```python
from build123d import *

# Parameters (mm, degrees)
BOSS_EXTRU_1_DEPTH = 10


with BuildPart() as part:
    # Esquisse1 → Boss.-Extru.1 (new body)
    with BuildSketch(Plane.XY):
        with BuildLine():
            Line((19.936371996, 9.53093454), (18.936003853, 6.945485686))
            ThreePointArc((18.936003853, 6.945485686), (18.933149277, 6.736662361), (19.067266911, 6.576575542))
            Line((19.067266911, 6.576575542), (21.475916438, 5.204099801))
            ThreePointArc((21.475916438, 5.204099801), (21.716214662, 4.879285253), (21.63795919, 4.482896797))
            Line((21.63795919, 4.482896797), (20.047921516, 2.211980154))
            ThreePointArc((20.047921516, 2.211980154), (19.995175197, 2.009908), (20.087084333, 1.822376562))
            Line((20.087084333, 1.822376562), (22.097287938, -0.08664509))
            ThreePointArc((22.097287938, -0.08664509), (22.252870323, -0.459528247), (22.082026846, -0.825670614))
            Line((22.082026846, -0.825670614), (19.994726852, -2.650077625))
            ThreePointArc((19.994726852, -2.650077625), (19.895154214, -2.833654908), (19.939513426, -3.03773232))
            Line((19.939513426, -3.03773232), (21.434445383, -5.372354483))
            ThreePointArc((21.434445383, -5.372354483), (21.496270047, -5.771635635), (21.242767367, -6.08625305))
            Line((21.242767367, -6.08625305), (18.779511342, -7.358122524))
            ThreePointArc((18.779511342, -7.358122524), (18.638899183, -7.512536093), (18.633130477, -7.72129924))
            Line((18.633130477, -7.72129924), (19.525910774, -10.345842161))
            ThreePointArc((19.525910774, -10.345842161), (19.490384691, -10.748316538), (19.168955462, -10.993124582))
            Line((19.168955462, -10.993124582), (16.472898893, -11.638540088))
            ThreePointArc((16.472898893, -11.638540088), (16.299419082, -11.754815988), (16.243857712, -11.956132315))
            Line((16.243857712, -11.956132315), (16.482601205, -14.718067098))
            ThreePointArc((16.482601205, -14.718067098), (16.351789022, -15.100344354), (15.981113543, -15.261115671))
            Line((15.981113543, -15.261115671), (13.208941437, -15.242568007))
            ThreePointArc((13.208941437, -15.242568007), (13.01267599, -15.313948704), (12.910550982, -15.496118438))
            Line((12.910550982, -15.496118438), (12.481382765, -18.234931474))
            ThreePointArc((12.481382765, -18.234931474), (12.262886811, -18.574795043), (11.864507393, -18.642186189))
            Line((11.864507393, -18.642186189), (9.177328317, -17.960753277))
            ThreePointArc((9.177328317, -17.960753277), (8.969683468, -17.983090385), (8.826929956, -18.135526484))
            Line((8.826929956, -18.135526484), (7.754791727, -20.692047914))
            ThreePointArc((7.754791727, -20.692047914), (7.461310193, -20.96974616), (7.0583792, -20.939840607))
            Line((7.0583792, -20.939840607), (4.612362234, -19.635124852))
            ThreePointArc((4.612362234, -19.635124852), (4.405405547, -19.607120219), (4.230319846, -19.720963651))
            Line((4.230319846, -19.720963651), (2.577520381, -21.946617741))
            ThreePointArc((2.577520381, -21.946617741), (2.226109347, -22.146011853), (1.842043663, -22.020547603))
            Line((1.842043663, -22.020547603), (-0.220657578, -20.168374341))
            ThreePointArc((-0.220657578, -20.168374341), (-0.414898532, -20.091655495), (-0.612141077, -20.160290093))
            Line((-0.612141077, -20.160290093), (-2.74954708, -21.925729918))
            ThreePointArc((-2.74954708, -21.925729918), (-3.138464883, -22.035231834), (-3.481344755, -21.821500413))
            Line((-3.481344755, -21.821500413), (-5.040853572, -19.529511222))
            ThreePointArc((-5.040853572, -19.529511222), (-5.211090216, -19.408536784), (-5.419026585, -19.427973754))
            Line((-5.419026585, -19.427973754), (-7.91682086, -20.630598369))
            ThreePointArc((-7.91682086, -20.630598369), (-8.320642942, -20.643844236), (-8.602410071, -20.354266937))
            Line((-8.602410071, -20.354266937), (-9.56809348, -17.755663898))
            ThreePointArc((-9.56809348, -17.755663898), (-9.704432278, -17.597464462), (-9.910977966, -17.566574199))
            Line((-9.910977966, -17.566574199), (-12.623997787, -18.136491432))
            ThreePointArc((-12.623997787, -18.136491432), (-13.019255477, -18.052711449), (-13.223534582, -17.704117452))
            Line((-13.223534582, -17.704117452), (-13.539270574, -14.949921928))
            ThreePointArc((-13.539270574, -14.949921928), (-13.633788011, -14.76369147), (-13.826939332, -14.684269203))
            Line((-13.826939332, -14.684269203), (-16.597513849, -14.588357536))
            ThreePointArc((-16.597513849, -14.588357536), (-16.961236207, -14.41242069), (-17.076155328, -14.025069012))
            Line((-17.076155328, -14.025069012), (-16.723594475, -11.275344836))
            ThreePointArc((-16.723594475, -11.275344836), (-16.770797541, -11.071906393), (-16.939329244, -10.948567856))
            Line((-16.939329244, -10.948567856), (-19.606442736, -10.192401327))
            ThreePointArc((-19.606442736, -10.192401327), (-19.91749154, -9.934532429), (-19.936371996, -9.53093454))
            Line((-19.936371996, -9.53093454), (-18.936003853, -6.945485686))
            ThreePointArc((-18.936003853, -6.945485686), (-18.933149277, -6.736662361), (-19.067266911, -6.576575542))
            Line((-19.067266911, -6.576575542), (-21.475916438, -5.204099801))
            ThreePointArc((-21.475916438, -5.204099801), (-21.716214662, -4.879285253), (-21.63795919, -4.482896797))
            Line((-21.63795919, -4.482896797), (-20.047921516, -2.211980154))
            ThreePointArc((-20.047921516, -2.211980154), (-19.995175197, -2.009908), (-20.087084333, -1.822376562))
            Line((-20.087084333, -1.822376562), (-22.097287938, 0.08664509))
            ThreePointArc((-22.097287938, 0.08664509), (-22.252870323, 0.459528247), (-22.082026846, 0.825670614))
            Line((-22.082026846, 0.825670614), (-19.994726852, 2.650077625))
            ThreePointArc((-19.994726852, 2.650077625), (-19.895154214, 2.833654908), (-19.939513426, 3.03773232))
            Line((-19.939513426, 3.03773232), (-21.434445383, 5.372354483))
            ThreePointArc((-21.434445383, 5.372354483), (-21.496270047, 5.771635635), (-21.242767367, 6.08625305))
            Line((-21.242767367, 6.08625305), (-18.779511342, 7.358122524))
            ThreePointArc((-18.779511342, 7.358122524), (-18.638899183, 7.512536093), (-18.633130477, 7.72129924))
            Line((-18.633130477, 7.72129924), (-19.525910774, 10.345842161))
            ThreePointArc((-19.525910774, 10.345842161), (-19.490384691, 10.748316538), (-19.168955462, 10.993124582))
            Line((-19.168955462, 10.993124582), (-16.472898893, 11.638540088))
            ThreePointArc((-16.472898893, 11.638540088), (-16.299419082, 11.754815988), (-16.243857712, 11.956132315))
            Line((-16.243857712, 11.956132315), (-16.482601205, 14.718067098))
            ThreePointArc((-16.482601205, 14.718067098), (-16.351789022, 15.100344354), (-15.981113543, 15.261115671))
            Line((-15.981113543, 15.261115671), (-13.208941437, 15.242568007))
            ThreePointArc((-13.208941437, 15.242568007), (-13.01267599, 15.313948704), (-12.910550982, 15.496118438))
            Line((-12.910550982, 15.496118438), (-12.481382765, 18.234931474))
            ThreePointArc((-12.481382765, 18.234931474), (-12.262886811, 18.574795043), (-11.864507393, 18.642186189))
            Line((-11.864507393, 18.642186189), (-9.177328317, 17.960753277))
            ThreePointArc((-9.177328317, 17.960753277), (-8.969683468, 17.983090385), (-8.826929956, 18.135526484))
            Line((-8.826929956, 18.135526484), (-7.754791727, 20.692047914))
            ThreePointArc((-7.754791727, 20.692047914), (-7.461310193, 20.96974616), (-7.0583792, 20.939840607))
            Line((-7.0583792, 20.939840607), (-4.612362234, 19.635124852))
            ThreePointArc((-4.612362234, 19.635124852), (-4.405405547, 19.607120219), (-4.230319846, 19.720963651))
            Line((-4.230319846, 19.720963651), (-2.577520381, 21.946617741))
            ThreePointArc((-2.577520381, 21.946617741), (-2.226109347, 22.146011853), (-1.842043663, 22.020547603))
            Line((-1.842043663, 22.020547603), (0.220657578, 20.168374341))
            ThreePointArc((0.220657578, 20.168374341), (0.414898532, 20.091655495), (0.612141077, 20.160290093))
            Line((0.612141077, 20.160290093), (2.74954708, 21.925729918))
            ThreePointArc((2.74954708, 21.925729918), (3.138464883, 22.035231834), (3.481344755, 21.821500413))
            Line((3.481344755, 21.821500413), (5.040853572, 19.529511222))
            ThreePointArc((5.040853572, 19.529511222), (5.211090216, 19.408536784), (5.419026585, 19.427973754))
            Line((5.419026585, 19.427973754), (7.91682086, 20.630598369))
            ThreePointArc((7.91682086, 20.630598369), (8.320642942, 20.643844236), (8.602410071, 20.354266937))
            Line((8.602410071, 20.354266937), (9.56809348, 17.755663898))
            ThreePointArc((9.56809348, 17.755663898), (9.704432278, 17.597464462), (9.910977966, 17.566574199))
            Line((9.910977966, 17.566574199), (12.623997787, 18.136491432))
            ThreePointArc((12.623997787, 18.136491432), (13.019255477, 18.052711449), (13.223534582, 17.704117452))
            Line((13.223534582, 17.704117452), (13.539270574, 14.949921928))
            ThreePointArc((13.539270574, 14.949921928), (13.633788011, 14.76369147), (13.826939332, 14.684269203))
            Line((13.826939332, 14.684269203), (16.597513849, 14.588357536))
            ThreePointArc((16.597513849, 14.588357536), (16.961236207, 14.41242069), (17.076155328, 14.025069012))
            Line((17.076155328, 14.025069012), (16.723594475, 11.275344836))
            ThreePointArc((16.723594475, 11.275344836), (16.770797541, 11.071906393), (16.939329244, 10.948567856))
            Line((16.939329244, 10.948567856), (19.606442736, 10.192401327))
            ThreePointArc((19.606442736, 10.192401327), (19.91749154, 9.934532429), (19.936371996, 9.53093454))
        make_face()
        with BuildLine():
            Line((14.953030626, -4.277181575), (16.501758042, -4.982426557))
            ThreePointArc((16.501758042, -4.982426557), (16.651785463, -5.134087079), (16.663083329, -5.347116418))
            ThreePointArc((16.663083329, -5.347116418), (15.924531384, -7.256672806), (14.968008895, -9.066901881))
            ThreePointArc((14.968008895, -9.066901881), (14.799864591, -9.198133844), (14.587009397, -9.184458985))
            Line((14.587009397, -9.184458985), (13.038282108, -8.478683252))
            ThreePointArc((13.038282108, -8.478683252), (12.832759155, -8.462847948), (12.665533258, -8.583371557))
            ThreePointArc((12.665533258, -8.583371557), (-13.922503409, 6.344596033), (14.787409001, -3.927153556))
            ThreePointArc((14.787409001, -3.927153556), (14.806182583, -4.132467854), (14.953030626, -4.277181575))
        make_face(mode=Mode.SUBTRACT)
    extrude(amount=BOSS_EXTRU_1_DEPTH)


solid = part.part
```
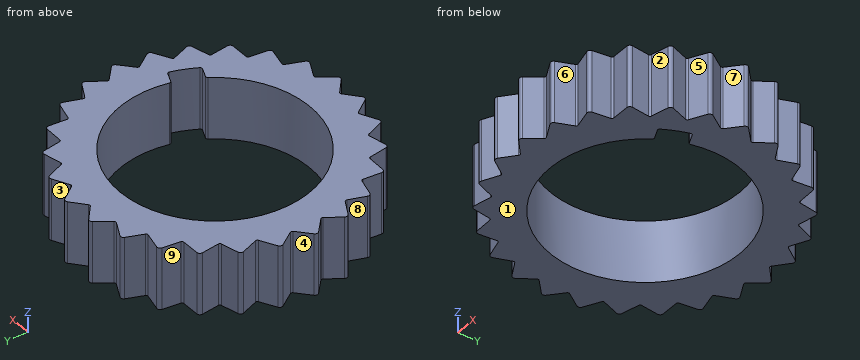
Could you check a few things on this model? Use its own coordinates, in mm. Face numbers are marked on the shaded views. A direction names the side the tool comes from. Coordinates: 2 decimals unless noted, no trailing zeros. Order: outer loops, then holes, each group sorted by start corner. A loop starts at its lowest first (then second) coordinate and runs counter-clockwise, first axis right, second up. Notation, with made-up numbers: M -34,-34 L 22,-34 A23 cw 22,-7 Z; hole C 41,-38.75 d3. An arc over 180 degrees is marked long. Use a Markdown table: item, result. Add a question column.
Q1. I'm going to push flat-ended pins straight in: pin 1 (1 mm diameter, centred on x = 4.5, z = 9, fed in from +Y); pin 2 (2 mm diameter, centred on y = -3.5, z = 5.5, fed in from +X); pin 3 (6 mm diameter, centred on x = 17.5, z = 4.5, fed in from +Y). Where does each tip first touch, or does it pass through?
Q2. I want a section at B-B on x = 11. List the corners of the cut face in (y, z) for me.
Q3. We'd pull the mould along Y, two halves only. Please class the marked faces 6, 7, 8 and 9: pulls with the +Y half, pulls with the -Y half, needs draft (parallel to the pull), parting line crosses it, or undercut.
Q4. If I drill on L1, parallel to Y at x = 0, z = 4.5; L2, parallel to X at y = 0.5, z = 5.5; L3, parallel to Y at x = 10, z = 8.25, over which ranges is the centre line in solid material (lowest first)?
Q5. I want a section at C-C on y = 16.5. List the corners of the cut face in (x, z) for me.
Q6. Which directions (+Z, -Z, +X, -X, +Y, -Y) give clear straight access to the entire face, cutting with the end or side of a thin tool? Please do the marked faces 1, 2, 3, 4 and 5.
Q7. I want a section at A-A on x = -6.5. List the corners of the cut face in (y, z) for me, then the cut area to 3 significant figures.
Checked values:
| question | item | result |
|---|---|---|
| 1 | pin 1 | y = 21.06 |
| 1 | pin 2 | x = 20.88 |
| 1 | pin 3 | y = 14.66 |
| 2 | outline | M -18.42,0 L -10.63,0 L -10.63,10 L -18.42,10 Z; M 10.63,0 L 17.8,0 L 17.8,10 L 10.63,10 Z |
| 3 | face 6 | pulls with the -Y half |
| 3 | face 7 | undercut |
| 3 | face 8 | undercut |
| 3 | face 9 | pulls with the +Y half |
| 4 | L1 | -20.37 to -15.3, 15.3 to 20.37 |
| 4 | L2 | -22.25 to -15.29, 15.29 to 21.48 |
| 4 | L3 | -18.17 to -11.58, 11.58 to 17.59 |
| 5 | outline | M -12.75,0 L 13.36,0 L 13.36,10 L -12.75,10 Z |
| 6 | face 1 | -Z, +X, -X, +Y, -Y |
| 6 | face 2 | +Z, -Z, +X, -Y |
| 6 | face 3 | +Z, -Z, +Y |
| 6 | face 4 | +Z, -Z, -X |
| 6 | face 5 | +Z, -Z, +X |
| 7 | outline | M -19.95,0 L -13.85,0 L -13.85,10 L -19.95,10 Z; M 13.85,0 L 20.64,0 L 20.64,10 L 13.85,10 Z |
| 7 | area | 129 mm² |
